```python
from build123d import *

# Parameters (mm, degrees)
SKETCH_230_R          = 7.3
EXTRUDE_254_DEPTH     = 0.5
SKETCH_305_R          = 10
EXTRUDE_323_DEPTH     = 4.6
SKETCH_364_W          = 4
SKETCH_364_H          = 4
EXTRUDE_412_DEPTH     = 0.5
SKETCH_471_W          = 0.267477204
SKETCH_471_H          = 0.791286728
SKETCH_471_W_2        = 0.261904762
SKETCH_471_H_2        = 2.691489362
SKETCH_471_W_3        = 0.490374874
SKETCH_471_H_3        = 3.722391084
SKETCH_471_W_4        = 0.373353597
SKETCH_471_H_4        = 2.59118541
CUT_EXTRUDE_814_DEPTH = 0.3


with BuildPart() as part:
    # Sketch 230 → Extrude 254 (new body)
    with BuildSketch(Plane.XY.offset(7.6)):
        with Locations((15, -35)):
            Circle(SKETCH_230_R)
    extrude(amount=EXTRUDE_254_DEPTH)

    # Sketch 305 → Extrude 323 (add)
    with BuildSketch(Plane.XY.offset(8.1)):
        with Locations((15, -35)):
            Circle(SKETCH_305_R)
    extrude(amount=EXTRUDE_323_DEPTH)

    # Sketch 364 → Extrude 412 (add)
    with BuildSketch(Plane.XY.offset(8.1)):
        with Locations((15, -24)):
            Rectangle(SKETCH_364_W, SKETCH_364_H)
    extrude(amount=EXTRUDE_412_DEPTH)

    # Sketch 471 → Cut-Extrude 814 (cut)
    # profile 1 of 6: a face of its own
    with BuildSketch(Plane.XY.offset(7.6)):
        Polygon((19.076241135, -35.76621074), (19.076241135, -33.793566363), (18.312816616, -33.793566363), (18.312816616, -33.386778116), (19.115248227, -33.386778116), (19.115248227, -32.72922999), (18.312816616, -32.72922999), (18.312816616, -32.25), (17.75, -32.25), (17.75, -32.72922999), (16.953140831, -32.72922999), (16.953140831, -33.386778116), (17.75, -33.386778116), (17.75, -33.793566363), (16.98100304, -33.793566363), (16.98100304, -35.76621074), (17.75, -35.76621074), (17.75, -36.156281662), (17.426798379, -35.877659574), (17.33407914, -35.968211753), (17.234239559, -36.068980074), (17.127279635, -36.179964539), (17.01319937, -36.301165147), (16.891998762, -36.432581898), (16.763677812, -36.574214792), (17.198328267, -36.98100304), (17.284855905, -36.871102105), (17.373550602, -36.760582011), (17.464412361, -36.649442756), (17.55744118, -36.537684341), (17.65263706, -36.425306766), (17.75, -36.31231003), (17.75, -37.738855117), (18.312816616, -37.738855117), (18.312816616, -36.529635258), (18.423646291, -36.723277609), (18.540667567, -36.910418777), (18.663880446, -37.091058764), (18.793284926, -37.265197568), (18.928881009, -37.432835191), (19.070668693, -37.593971631), (19.117570078, -37.471997073), (19.165400203, -37.351260835), (19.214159068, -37.231762918), (19.263846673, -37.113503321), (19.314463019, -36.996482044), (19.366008105, -36.880699088), (19.200227964, -36.729004841), (19.040949004, -36.563689069), (18.888171226, -36.384751773), (18.74189463, -36.192192953), (18.602119216, -35.986012608), (18.468844985, -35.76621074), align=None)
        with Locations((17.616261398, -34.779888551)):
            Rectangle(SKETCH_471_W, SKETCH_471_H, mode=Mode.SUBTRACT)
        with Locations((18.443768997, -34.779888551)):
            Rectangle(SKETCH_471_W_2, SKETCH_471_H, mode=Mode.SUBTRACT)
    # profile 2 of 6: a face of its own
    with BuildSketch(Plane.XY.offset(7.6)):
        Polygon((19.260131712, -32.640070922), (19.260131712, -36.590932118), (20.023556231, -36.590932118), (20.023556231, -37.153748734), (20.541793313, -37.153748734), (20.541793313, -32.640070922), align=None)
        with Locations((19.889817629, -34.61550152)):
            Rectangle(SKETCH_471_W, SKETCH_471_H_2, mode=Mode.SUBTRACT)
    # profile 3 of 6: a face of its own
    with BuildSketch(Plane.XY.offset(7.6)):
        Polygon((16.000253293, -32.25), (15.426291793, -32.25), (15.426291793, -37.020010132), (15.442544748, -37.211485422), (15.491303614, -37.369835641), (15.572568389, -37.49506079), (15.686339075, -37.587160869), (15.83261567, -37.646135878), (16.011398176, -37.671985816), (16.735815603, -37.671985816), (16.749127547, -37.546760666), (16.763058651, -37.427417539), (16.777608916, -37.313956434), (16.792778341, -37.20637735), (16.808566926, -37.104680288), (16.824974671, -37.008865248), (16.750056287, -37.017688281), (16.670184622, -37.025582573), (16.585359676, -37.032548126), (16.495581448, -37.038584938), (16.400849938, -37.043693009), (16.301165147, -37.04787234), (16.209219858, -37.040442418), (16.133991895, -37.018152651), (16.075481256, -36.98100304), (16.033687943, -36.928993583), (16.008611955, -36.862124282), (16.000253293, -36.780395137), align=None)
    # profile 4 of 6: a face of its own
    with BuildSketch(Plane.XY.offset(7.6)):
        with Locations((16.512917933, -34.646149949)):
            Rectangle(SKETCH_471_W_3, SKETCH_471_H_3)
    # profile 5 of 6: a face of its own
    with BuildSketch(Plane.XY.offset(7.6)):
        Polygon((14.835612969, -32.595491388), (13.102583587, -32.595491388), (13.102583587, -36.323454914), (12.916061578, -35.878123945), (12.765141281, -35.355707531), (12.649822695, -34.756205674), (12.57010582, -34.079618372), (12.525990656, -33.325945626), (12.517477204, -32.495187437), (11.804204661, -32.556484296), (11.804204661, -33.084318361), (11.815349544, -33.583051897), (11.837639311, -34.052684904), (11.871073961, -34.493217382), (11.915653495, -34.90464933), (11.971377913, -35.28698075), (12.065799842, -35.743920973), (12.189322301, -36.18228639), (12.341945289, -36.602077001), (12.523668806, -37.003292806), (12.734492852, -37.385933806), (12.974417427, -37.75), (13.039274457, -37.671676236), (13.118681752, -37.581588427), (13.212639311, -37.479736575), (13.321147135, -37.36612068), (13.444205223, -37.240740741), (13.581813576, -37.103596758), (13.500084431, -36.991219183), (13.422070247, -36.876984127), (13.347771023, -36.760891591), (13.277186761, -36.642941574), (13.21031746, -36.523134076), (13.147163121, -36.401469098), (14.155775076, -36.401469098), (14.155775076, -36.752532928), (14.835612969, -36.752532928), align=None)
        with Locations((13.969098278, -34.498480243)):
            Rectangle(SKETCH_471_W_4, SKETCH_471_H_4, mode=Mode.SUBTRACT)
    # profile 6 of 6: a face of its own
    with BuildSketch(Plane.XY.offset(7.6)):
        Polygon((10.511398176, -32.34473151), (10.494526061, -33.312478892), (10.414190026, -34.194782168), (10.270390071, -34.991641337), (10.063126196, -35.7030564), (9.792398401, -36.329027356), (9.458206687, -36.869554205), (9.548449285, -36.996017674), (9.640858944, -37.126505685), (9.735435664, -37.261018237), (9.832179444, -37.39955533), (9.931090285, -37.542116965), (10.032168186, -37.688703141), (10.407379264, -37.041990319), (10.712006079, -36.301784307), (10.946048632, -35.468085106), (11.109506923, -34.540892716), (11.202380952, -33.520207137), (11.224670719, -32.406028369), align=None)
    extrude(amount=CUT_EXTRUDE_814_DEPTH, mode=Mode.SUBTRACT)


solid = part.part
```
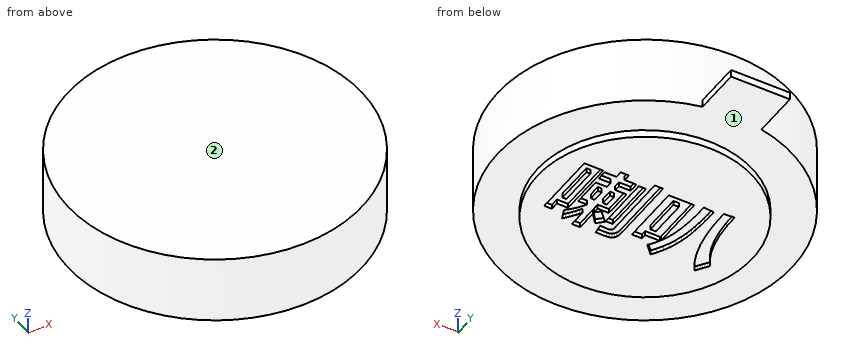
Check sheet for the modelled part. Datum: model origin and axes. Units: mm. Face numbers are marked on the shaded views. A direction names the side the tool comes from. Round coordinates to 2 decimals unless told otherwise and drop trailing zeros. Order: outer loops, then holes, each group sorted by start corner. A loop starts at its lowest first (then second) coordinate and runs counter-clockwise, first axis right, second up. Notation, with made-up numbers: (19.25, -11) - (76.25, -11) arc R22 ccw to (76.25, 0) - close; hole circle Ø5 at (18.5, 25.5). An arc over 180 degrees is marked (long way). Write item = value, one per line.
Q1. Section check B-B (y = -41.5). Record the boundary of the cut face in (x, z), and give its area (3 significant figures).
Computed:
outline = (7.4, 8.1) - (11.68, 8.1) - (11.68, 7.6) - (18.32, 7.6) - (18.32, 8.1) - (22.6, 8.1) - (22.6, 12.7) - (7.4, 12.7) - close
area = 73.2 mm^2
Q2. Section check C-C (z = 12). Record the boundary of the cut face in (x, y).
Computed:
outline = circle Ø20 at (15, -35)
Q3. Tool access check on the marked faces 1 and 2. Record the directions out of +Z, -Z, +X, -X, +Y, -Y that give a thin tool (end or side, any length) a straight path to the whole face; none if there is none.
Computed:
face_1 = -Z
face_2 = +Z, +X, -X, +Y, -Y
Q4. Section check D-D (y = -25.5). Record the boundary of the cut face in (x, z).
Computed:
outline = (11.88, 8.1) - (18.12, 8.1) - (18.12, 12.7) - (11.88, 12.7) - close
Q5. Thickness scan on line 1 along Z through (x, y) = (7.75, -33.25); line 2 along Z through (x, y) = (16.5, -34.25); line 3 along X through (y, z) = (-24.75, 8.45). Record the ranges inside material, lowest first.
Computed:
line_1 = 8.1 to 12.7
line_2 = 7.9 to 12.7
line_3 = 13 to 17
Q6. Go/stop test with flat-tipped pins: pin 1 (2 mm diameter, centred on y = -38, z = 8, fed in from +X); pin 2 (1 mm diameter, centred on y = -39, z = 11.5, fed in from +X). Record where each tip stops, or that it passes through.
Computed:
pin_1 = 24.8
pin_2 = 24.37
Q7. Section check A-A (z = 8.35). Record the boundary of the cut face in (x, y), and give its area (3 significant figures).
Computed:
outline = (13, -25.2) arc R10 ccw (long way) to (17, -25.2) - (17, -22) - (13, -22) - close
area = 326 mm^2
